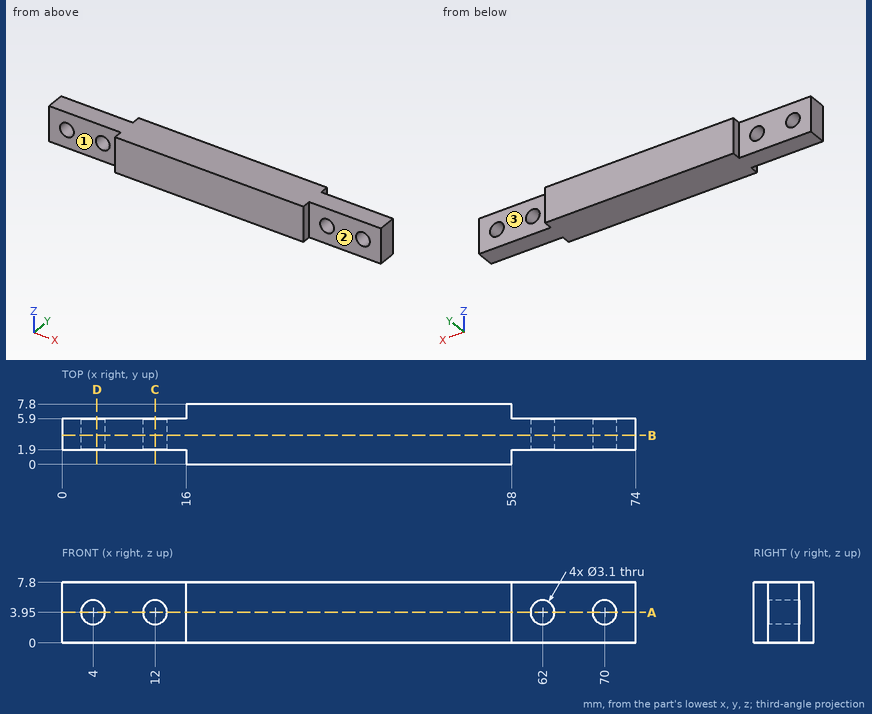
Study the drawing (mm; zero at the part's minimum x, y, z) and answer. A direction names the side the tool comes from. Give positions to 0.01 mm unless a question says otherwise; leave off trailing zeros. Write each loop counter-clockwise with the first axis right and the second up, starting at its lowest first coordinate (ties: lowest second). Pieces come first, ordered by that corner, then holes.
(1) Which of the six approach directions +Z, -Z, +X, -X, +Y, -Y give full straight-line access (tool end or side, diameter ignored) to the marked faces 1, 2 and 3?
Final values:
face 1: +Z, -Z, -X, -Y
face 2: +Z, -Z, +X, -Y
face 3: +Z, -Z, +X, +Y
(2) The part is cut by section D-D on x = 4.5. Write down the section's boundary in (y, z).
Final values:
outline: (1.9, 0) - (5.9, 0) - (5.9, 2.48) - (1.9, 2.48) - close; (1.9, 5.42) - (5.9, 5.42) - (5.9, 7.8) - (1.9, 7.8) - close
(3) The part is cut by section B-B on y = 3.75. Write down the section's boundary in (x, z).
Final values:
outline: (0, 0) - (74, 0) - (74, 7.8) - (0, 7.8) - close; hole circle Ø3.1 at (4, 3.95); hole circle Ø3.1 at (12, 3.95); hole circle Ø3.1 at (62, 3.95); hole circle Ø3.1 at (70, 3.95)
(4) The part is cut by section A-A on z = 3.95. Write down the section's boundary in (x, y).
Final values:
outline: (0, 1.9) - (2.45, 1.9) - (2.45, 5.9) - (0, 5.9) - close; (5.55, 1.9) - (10.45, 1.9) - (10.45, 5.9) - (5.55, 5.9) - close; (13.55, 1.9) - (16, 1.9) - (16, 0) - (58, 0) - (58, 1.9) - (60.45, 1.9) - (60.45, 5.9) - (58, 5.9) - (58, 7.8) - (16, 7.8) - (16, 5.9) - (13.55, 5.9) - close; (63.55, 1.9) - (68.45, 1.9) - (68.45, 5.9) - (63.55, 5.9) - close; (71.55, 1.9) - (74, 1.9) - (74, 5.9) - (71.55, 5.9) - close
(5) Straight lines are drawn through the part: line 1 (X direction, y = 3, z = 4); line 2 (Z direction, x = 62, y = 3.5); line 3 (X direction, y = 5.75, z = 3). For each, find the intervals that lie inside material, in ascending order.
Final values:
line 1: x = 0 to 2.45, 5.55 to 10.45, 13.55 to 60.45, 63.55 to 68.45, 71.55 to 74
line 2: z = 0 to 2.4, 5.5 to 7.8
line 3: x = 0 to 2.78, 5.22 to 10.78, 13.22 to 60.78, 63.22 to 68.78, 71.22 to 74
(6) Flat-ended cylindrical pins translate along their axes: pin 1 Ø0.6 at (y, z) = (6.5, 3.5) entering from -X; pin 2 Ø4 at (x, z) = (65, 3) entering from +Y; pin 3 Ø4 at (x, z) = (9, 5.5) entering from -Y. Find the tip coordinate at first contact, or state that the pin passes through.
Final values:
pin 1: stops at x = 16
pin 2: stops at y = 5.9
pin 3: stops at y = 1.9
(7) The part is cut by section C-C on x = 12. Write down the section's boundary in (y, z).
Final values:
outline: (1.9, 0) - (5.9, 0) - (5.9, 2.4) - (1.9, 2.4) - close; (1.9, 5.5) - (5.9, 5.5) - (5.9, 7.8) - (1.9, 7.8) - close
